For this review, take the finished solid that the model builds, in its own axes (mm). Face numbers are marked on the shaded views. A direction names the side the tool comes from. Round coordinates to 2 decimals unless told otherwise and drop trailing zeros. Put each result on its own line as item: value.
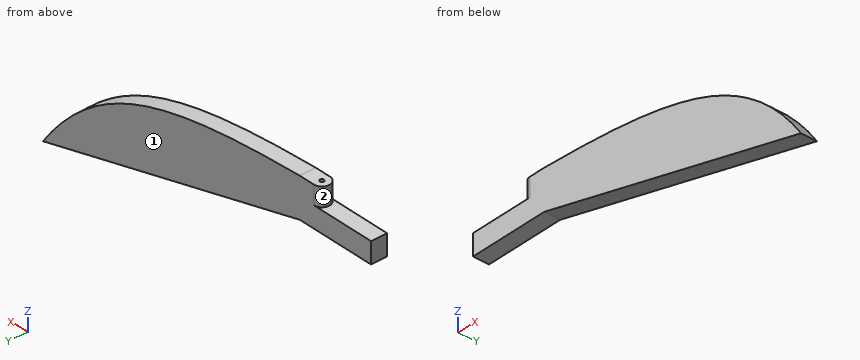
from build123d import *

# Parameters (mm, degrees)
SALIENTE_EXTRUIR1_DEPTH = 5
CROQUIS3_W              = 12.5
CROQUIS3_H              = 5
SALIENTE_EXTRUIR2_DEPTH = 25
CROQUIS6_R              = 0.63
CORTAR_EXTRUIR3_DEPTH   = 1.5
CORTAR_EXTRUIR4_DEPTH   = 5.875


with BuildPart() as part:
    # Croquis2 → Saliente-Extruir1 (new body)
    with BuildSketch(Plane(origin=(0, 0, 0), x_dir=(1, 0, 0), z_dir=(0, 1, 0))):
        with BuildLine():
            Line((0, 0), (0, 12.5))
            Line((0, 12.5), (90, 35.865427318))
            add(Edge.make_bspline(
                [(0, 0), (0.394136999, 0.015797336), (1.194952966, 0.048834045), (2.992448828, 0.125211317), (4.579856068, 0.200911656), (6.612637351, 0.301249971), (8.392251736, 0.398752477), (10.315878033, 0.509903005), (12.159048858, 0.626310038), (14.511736704, 0.785189542), (17.305717547, 0.994336582), (20.114398042, 1.2314722), (22.909905137, 1.499776667), (25.707540494, 1.796493489), (29.430521004, 2.232380684), (34.457318955, 2.928516321), (39.917638309, 3.8880509), (45.326966885, 5.105084916), (49.769918493, 6.319079443), (53.346159155, 7.448006204), (56.870231766, 8.730995456), (60.329622828, 10.180098556), (63.710264837, 11.804910517), (66.997597592, 13.611491814), (70.17732587, 15.601579919), (72.854283587, 17.500893709), (75.067204078, 19.237089159), (76.854732505, 20.752585132), (78.250168573, 22.004629224), (79.619707974, 23.303249768), (80.962355597, 24.647453618), (82.277321506, 26.036087115), (83.403178931, 27.288894321), (84.345387571, 28.382707102), (85.115533062, 29.306902867), (85.722715368, 30.053623655), (86.321025458, 30.807421985), (86.910712224, 31.56828047), (87.491255325, 32.335040025), (88.06431213, 33.109755161), (88.629936117, 33.892108149), (89.099903233, 34.555740193), (89.55695597, 35.215829282), (89.829292977, 35.613909175), (89.943246974, 35.781569234), (90, 35.865427318)],
                knots=[0.074822974, 0.074822974, 0.074822974, 0.074822974, 0.074822974, 0.090398408, 0.105973841, 0.121549274, 0.137124708, 0.152700141, 0.168275574, 0.183851007, 0.199426441, 0.230577307, 0.261728173, 0.277303606, 0.29287904, 0.324029906, 0.386331636, 0.445924571, 0.477075434, 0.508226306, 0.539377159, 0.57052801, 0.601678868, 0.632829681, 0.663980451, 0.695131352, 0.726282194, 0.741857688, 0.757433182, 0.773008671, 0.788584161, 0.804576906, 0.820569651, 0.836562506, 0.844558934, 0.852555362, 0.860551891, 0.86854842, 0.87654495, 0.884541479, 0.89253801, 0.900534541, 0.908531072, 0.912529338, 0.916527603, 0.916527603, 0.916527603, 0.916527603, 0.916527603], degree=4))
        make_face()
    extrude(amount=SALIENTE_EXTRUIR1_DEPTH)

    # Croquis3 → Saliente-Extruir2 (add)
    with BuildSketch(Plane.ZY):
        with Locations((-6.25, 2.5)):
            Rectangle(CROQUIS3_W, CROQUIS3_H)
    extrude(amount=SALIENTE_EXTRUIR2_DEPTH)

    # Croquis6 → Cortar-Extruir3 (cut)
    with BuildSketch(Plane.XY):
        with Locations((-5, 2.5)):
            Circle(CROQUIS6_R)
    extrude(amount=-CORTAR_EXTRUIR3_DEPTH, mode=Mode.SUBTRACT)

    # Croquis5 → Cortar-Extruir4 (cut)
    with BuildSketch(Plane.XY):
        with BuildLine():
            Line((-25, 5), (-25, 0))
            Line((-25, 0), (-4.999999991, 0))
            ThreePointArc((-4.999999991, 0), (-7.5, 2.499999995), (-5, 5))
            Line((-5, 5), (-25, 5))
        make_face()
    extrude(amount=-CORTAR_EXTRUIR4_DEPTH, mode=Mode.SUBTRACT)


solid = part.part
(1) To check wall thickness, follow L1, parallel to Z at x = -9.5, y = 0.25 (3 decimals); L2, parallel to Z at x = -2.5, y = 2.9. State the ranges of each line that lie inside material, in increasing order.
A:
L1: z = -12.5 to -5.875
L2: z = -12.5 to 0
(2) Insertion check: pin 1 Ø8 at (x, z) = (51, -15.5) entering from -Y; pin 2 Ø3 at (y, z) = (1.5, -23) entering from +X; pin 3 Ø0.8 at (x, y) = (-5, 2.5) entering from +Z; pin 4 Ø1.5 at (x, y) = (-15.5, 2) entering from +Z (3 decimals). Each pin has a flat end and moves straight along its axis. Give the tip position at first contact, or say it passes through.
A:
pin 1: stops at y = 0
pin 2: stops at x = 80.8
pin 3: stops at z = -1.5
pin 4: stops at z = -5.875
(3) For the marked faces 1 and 2, list the 3-axis set-ups (+Z, -Z, +X, -X, +Y, -Y) from which the entire face can be reached by the end or side of a thin tool; tool diameter is ignored.
A:
face 1: +Z, -Z, +X, -X, +Y
face 2: +Z, -X
